Can you work these out from the drawing? Everything is in mm from the part's minimum corner. A direction names the side the tool comes from. Round coordinates to 2 decimals unless told otherwise and drop trailing zeros. Write each loop counter-clockwise with the first axis right and the second up, starting at its lowest first coordinate (ties: lowest second). Pieces come first, ordered by that corner, then holes. Notation, with made-up numbers: (43.5, 6) - (48.5, 6) arc R30 cw to (48.5, 34) - close; hole circle Ø6 at (88.25, 23). An arc over 180 degrees is marked (long way). One line per item, written item: value. Start each with the question number.
(1) I'm going to push flat-ended pins straight in: pin 1 Ø3 at (x, y) = (11, 28) entering from +Z; pin 2 Ø12 at (x, z) = (9, 20) entering from +Y; pin 3 Ø1 at (x, z) = (4.5, 23.5) entering from +Y; pin 4 Ø2 at (x, y) = (19.5, 40) entering from -Z. Where does each tip first touch, or does it pass through?
(2) I want a section at C-C on x = 20. List the corners of the cut face in (y, z) for me, plus the area to 4 significant figures.
(3) I want a section at D-D on z = 46.5. List the corners of the cut face in (x, y) for me, plus the area to 3 significant figures.
(4) Thinking about a two-plate mould opening in X: for the marked faces 4, 5 and 6, which applies, +X half, -X half, draft (parallel to the pull), parting line (faces both ways), or undercut?
(5) I want a section at B-B on y = 33. List the corners of the cut face in (x, z) for me.
(6) I want a section at A-A on z = 27. List the corners of the cut face in (x, y) for me, plus the area to 3 significant figures.
(7) If I drill on L1, parallel to Y at x = 20, z = 17; L2, parallel to Y at x = 8, z = 16; L3, parallel to Z at x = 13, y = 30.5, over which ranges is the centre line in solid material (lowest first)? Write a range as from..to.
(8) On a 3-axis mill with a long thin cutter (end or side, diameter ignored), from which of +Z, -Z, +X, -X, +Y, -Y can I reach the whole of each face in a straight line? I mean the marked faces 1, 2 and 3. Say none if no direction works.
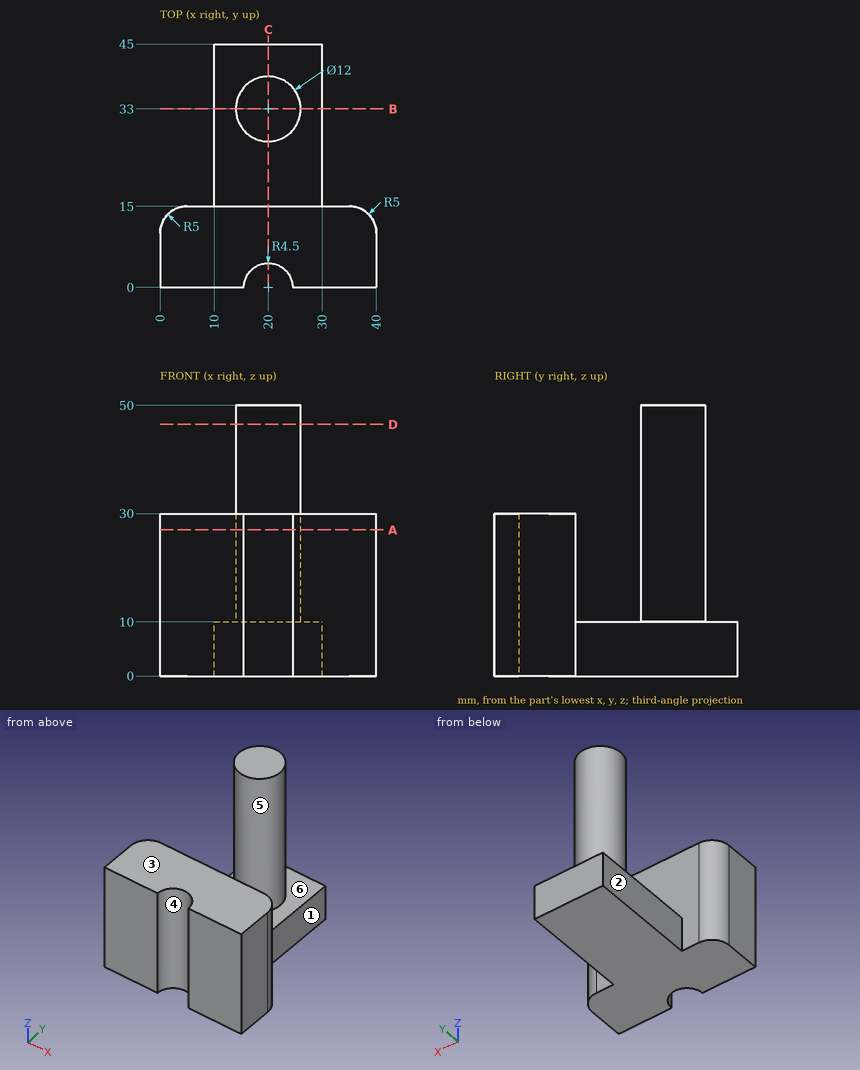
Established:
1. pin 1: z = 10
1. pin 2: y = 36.32
1. pin 3: y = 15
1. pin 4: z = 0
2. outline: (4.5, 0) - (45, 0) - (45, 10) - (39, 10) - (39, 50) - (27, 50) - (27, 10) - (15, 10) - (15, 30) - (4.5, 30) - close
2. area: 1,095 mm2
3. outline: circle Ø12 at (20, 33)
3. area: 113 mm2
4. face 4: undercut
4. face 5: parting line
4. face 6: draft
5. outline: (10, 0) - (30, 0) - (30, 10) - (26, 10) - (26, 50) - (14, 50) - (14, 10) - (10, 10) - close
6. outline: (0, 0) - (15.5, 0) arc R4.5 cw to (24.5, 0) - (40, 0) - (40, 10) arc R5 ccw to (35, 15) - (5, 15) arc R5 ccw to (0, 10) - close; circle Ø12 at (20, 33)
6. area: 671 mm2
7. L1: 4.5..15, 27..39
7. L2: 0..15
7. L3: 0..10
8. face 1: +Z, -Z, +X, +Y
8. face 2: +Z, -Z, -X, +Y
8. face 3: +Z, +X, -X, -Y
